from build123d import *

# Parameters (mm, degrees)
SKETCH_1_W      = 250
SKETCH_1_H      = 28.996988848
EXTRUDE_1_DEPTH = 8
SKETCH_2_W      = 21.001828318
SKETCH_2_H      = 4.50112507
EXTRUDE_2_DEPTH = 5.5
SKETCH_3_W      = 20.998493162
SKETCH_3_H      = 4.496055774
EXTRUDE_3_DEPTH = 5.5


with BuildPart() as part:
    # Эскиз1 → Бобышка-Вытянуть1 (new body)
    with BuildSketch(Plane(origin=(0, 0, 0), x_dir=(1, 0, 0), z_dir=(0, 1, 0))):
        Rectangle(SKETCH_1_W, SKETCH_1_H)
    extrude(amount=EXTRUDE_1_DEPTH)

    # Эскиз2 → Бобышка-Вытянуть2 (add)
    with BuildSketch(Plane(origin=(125, 0, 0), x_dir=(0, 0, -1), z_dir=(1, 0, 0))):
        with Locations((0, 4)):
            Rectangle(SKETCH_2_W, SKETCH_2_H)
    extrude(amount=EXTRUDE_2_DEPTH)

    # Эскиз3 → Бобышка-Вытянуть3 (add)
    with BuildSketch(Plane.ZY.offset(125)):
        with Locations((0, 4)):
            Rectangle(SKETCH_3_W, SKETCH_3_H)
    extrude(amount=EXTRUDE_3_DEPTH)


solid = part.part
CAD build for the part. Positions are in the model's coordinates, mm. A direction names the side the tool comes from. Give positions to 0.01 mm unless a question says otherwise; leave off trailing zeros. Write each loop counter-clockwise with the first axis right and the second up, starting at its lowest first coordinate (ties: lowest second). Pieces come first, ordered by that corner, then holes. Notation, with made-up numbers: M 60,78 L 85,78 A20 ccw 85,84 Z; hole C 2,41.5 d4. An arc over 180 degrees is marked long. Put each result on its own line as item: value. Start each with the question number.
(1) Probe L1, parallel to X at y = 6.75, z = -2.5. List the from-to ranges inside material, lowest first.
(2) Flat gauge pins, fed straight in: pin 1 Ø1.3 at (x, y) = (-128, 4.5) entering from +Z; pin 2 Ø4.5 at (x, z) = (127.5, 5) entering from -Y; pin 3 Ø1.6 at (x, z) = (127, -1) entering from +Y. Where does each tip first touch, or does it go through?
(3) Which spindle directions (+Z, -Z, +X, -X, +Y, -Y) get a long thin tool onto all of the face, cutting with end or side? Do faces 1 (the face through (-128, 4, -10.499)), 2 (the face through (-128, 1.752, 0)), 3 (the face through (128, 6.251, 0)). Say none if no direction does.
(4) Band-saw the part on A-A, the plane z = -3. Write the cut outline in (x, y), and give its area (3 significant figures).
Response values:
1. L1: x = -125 to 125
2. pin 1: stops at z = 10.5
2. pin 2: stops at y = 1.75
2. pin 3: stops at y = 6.25
3. face 1: -Z, -X, +Y, -Y
3. face 2: +Z, -Z, -X, -Y
3. face 3: +Z, -Z, +X, +Y
4. outline: M -130.5,1.75 L -125,1.75 L -125,0 L 125,0 L 125,1.75 L 130.5,1.75 L 130.5,6.25 L 125,6.25 L 125,8 L -125,8 L -125,6.25 L -130.5,6.25 Z
4. area: 2,050 mm2
